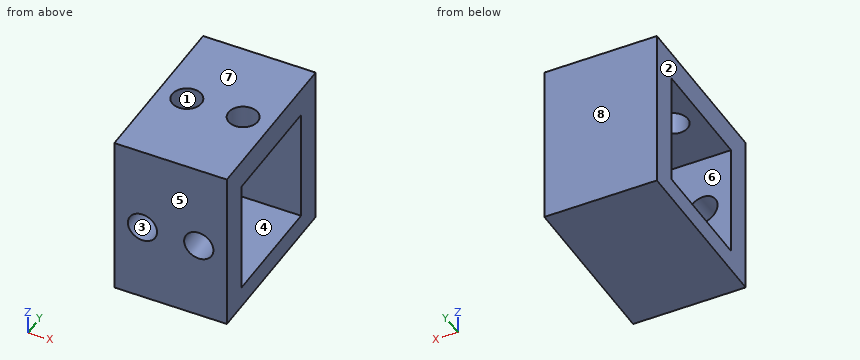
Autodesk Fusion 360 part; units mm, degrees
sketch "스케치1" plane through (0, 0, 0) normal (1, 0, 0) x (0, 1, 0)
  line L0 (15.2, 15.2) -> (-15.2, 15.2)
  line L1 (-15.2, 15.2) -> (-15.2, -15.2)
  line L2 (-15.2, -15.2) -> (15.2, -15.2)
  line L3 (15.2, -15.2) -> (15.2, 15.2)
  line L4 (15.2, 15.2) -> (-15.2, -15.2) construction
  line L5 (-15.2, 15.2) -> (15.2, -15.2) construction
  line L6 (10.2, 10.2) -> (-10.2, 10.2)
  line L7 (-10.2, 10.2) -> (-10.2, -10.2)
  line L8 (-10.2, -10.2) -> (10.2, -10.2)
  line L9 (10.2, -10.2) -> (10.2, 10.2)
  line L10 (10.2, 10.2) -> (-10.2, -10.2) construction
  line L11 (-10.2, 10.2) -> (10.2, -10.2) construction
  dimension "d1" = 30.4
  dimension "d2" = 30.4
  dimension "d3" = 20.4
  dimension "d4" = 20.4
extrude "돌출1" add sketch "스케치1" along normal blind 20
extrude "돌출2" cut 1 faces at (13.3333, -5.0667, -15.2) along direction (0, 0, 1) blind 1.2
sketch "스케치2" plane through (0, 0, 15.2) normal (0, 0, 1) x (-1, 0, 0)
  line L0 (0, -15.2) -> (0, 15.2)
  line L1 (0, 15.2) -> (-20, 15.2)
  line L2 (-20, 15.2) -> (-20, -15.2)
  line L3 (-20, -15.2) -> (0, -15.2)
  line L4 (0, 0) -> (-5, 0)
  circle A0 centre (-5, 0) radius 2.6
  line L5 (-20, 0) -> (-15, 0)
  circle A1 centre (-15, 0) radius 2.6
  dimension "d9" = 5
  dimension "d10" = 5.2
  dimension "d11" = 5
  dimension "d12" = 5.2
extrude "돌출3" cut sketch "스케치2" against normal blind 10 contours A0 | A1
sketch "스케치3" plane through (0, -15.2, 0) normal (0, -1, 0) x (1, 0, 0)
  line L0 (0, -14) -> (20, -14)
  line L1 (20, -14) -> (20, 15.2)
  line L2 (20, 15.2) -> (0, 15.2)
  line L3 (0, 15.2) -> (0, -14)
  line L4 (0, 0) -> (5, 0)
  line L5 (20, 0) -> (15, 0)
  circle A0 centre (5, 0) radius 2.6
  circle A1 centre (15, 0) radius 2.6
  dimension "d15" = 5
  dimension "d16" = 5
  dimension "d17" = 5.2
  dimension "d18" = 5.2
extrude "돌출4" cut sketch "스케치3" against normal blind 5 contours A1 | A0
Design review of the part built by this model. Coordinates are the model's own, in mm. Face numbers are marked on the shaded views. A direction names the side the tool comes from. Give positions to 0.01 mm unless a question says otherwise; leave off trailing zeros. Loops run counter-clockwise (first coordinate to the right, second up) from the corner with the lowest first, then second, coordinate; pieces in that order, holes last. Notation, with made-up numbers: (82.5, 1) -> (129.5, 1) arc R17 cw to (129.5, 26) -> close; hole circle Ø8 at (-34.5, 41). An arc over 180 degrees is marked (long way). One line per item, written item: value.
Q1. We need section A-A on z = 4.25. Give the boundary of the cut face in (x, y).
Numbers:
outline: (0, -15.2) -> (20, -15.2) -> (20, -10.2) -> (0, -10.2) -> close; (0, 10.2) -> (20, 10.2) -> (20, 15.2) -> (0, 15.2) -> close
Q2. Machinability: for the marked faces 1, 2, 3, 4 and 5, which of the approach directions +Z, -Z, +X, -X, +Y, -Y give a long, thin tool a straight path to every point of the face, cutting with its end or side? Answer none if there is none.
Numbers:
face 1: +Z
face 2: +Z, -Z, -X, +Y, -Y
face 3: -Y
face 4: +X, -X
face 5: +Z, -Z, +X, -X, -Y
Q3. We need section B-B on x = 2. Give the boundary of the cut face in (y, z).
Numbers:
outline: (-15.2, -14) -> (15.2, -14) -> (15.2, 15.2) -> (-15.2, 15.2) -> close; hole (-10.2, -10.2) -> (10.2, -10.2) -> (10.2, 10.2) -> (-10.2, 10.2) -> close
Q4. We need section D-D on z = 0. Give the boundary of the cut face in (x, y).
Numbers:
outline: (0, -15.2) -> (2.4, -15.2) -> (2.4, -10.2) -> (0, -10.2) -> close; (0, 10.2) -> (20, 10.2) -> (20, 15.2) -> (0, 15.2) -> close; (7.6, -15.2) -> (12.4, -15.2) -> (12.4, -10.2) -> (7.6, -10.2) -> close; (17.6, -15.2) -> (20, -15.2) -> (20, -10.2) -> (17.6, -10.2) -> close
Q5. We need section C-C on y = -3. Give the boundary of the cut face in (x, z), and give its area (3 significant figures).
Numbers:
outline: (0, -14) -> (20, -14) -> (20, -10.2) -> (0, -10.2) -> close; (0, 10.2) -> (20, 10.2) -> (20, 15.2) -> (0, 15.2) -> close
area: 176 mm^2
Q6. Draft analysis for pull direction Y (two halves, no side actions). For the marked faces 6, 7 and 8, state which applies: pulls with the +Y half, pulls with the -Y half, needs draft (parallel to the pull), parting line crosses it, or undercut.
Numbers:
face 6: undercut
face 7: needs draft
face 8: pulls with the +Y half
Q7. For L1, parallel to Y at x = 5, z = 13.55; L2, parallel to Y at x = 13, z = -7.5; L3, parallel to X at y = 0, z = 13.3, list the stretches that pass through material, from the lowest coordinate up.
Numbers:
L1: y = -15.2 to -2.6, 2.6 to 15.2
L2: y = -15.2 to -10.2, 10.2 to 15.2
L3: x = 0 to 2.4, 7.6 to 12.4, 17.6 to 20
Q8. For pin 1 Ø1 at (x, z) = (3, 0.5) entering from -Y, flat-tipped, find the tip position at first contact; note if it passes through.
Numbers:
pin 1: stops at y = 10.2
